```python
from build123d import *

# Parameters (mm, degrees)
F0_W           = 20.32
F0_H           = 12.7
F1_DEPTH       = 37.084
F5_D           = 9.525
F5_DEPTH       = 6.35
F5_TIP         = 2.8615986981
F5_ON_F3_D     = 9.525
F5_ON_F3_DEPTH = 6.35
F5_ON_F3_TIP   = 2.8615986981
F5_ON_F4_D     = 9.525
F5_ON_F4_DEPTH = 6.35
F5_ON_F4_TIP   = 2.8615986981
F7_DEPTH       = 37.085
F8_R           = 5.08


# Not quite as in the source:
# - a length typed as a fraction of an inch, garbled in the dataset ("3 / 203.2 mm" for 3/8 in), is restored


with BuildPart() as f1:
    # F0 (on Top) → F1 (new body)
    with BuildSketch(Plane.XY):
        with Locations((58.5882579065, 69.85)):
            Rectangle(F0_W, F0_H)
        Polygon((48.4282579065, 63.5), (-36.6617420935, 63.5), (0, 0), (117.1765158129, 0), (153.8382579065, 63.5), (68.7482579065, 63.5), align=None)
    extrude(amount=F1_DEPTH)

    # F5
    with Locations(Plane(origin=(0, 63.5, 0), x_dir=(-1, 0, 0), z_dir=(0, 1, 0))):
        with Locations((-136.8202579065, 18.542), (-119.8022579065, 18.542), (-102.7842579065, 18.542), (-85.7662579065, 18.542)):
            Hole(F5_D / 2, depth=F5_DEPTH)
            with Locations((0, 0, -(F5_DEPTH + F5_TIP / 2))):  # 118° drill point
                Cone(0, F5_D / 2, F5_TIP, mode=Mode.SUBTRACT)

    # F5 on F3
    with Locations(Plane(origin=(0, 63.5, 0), x_dir=(-1, 0, 0), z_dir=(0, 1, 0))):
        with Locations((-31.4102579065, 18.542), (-14.3922579065, 18.542), (2.6257420935, 18.542), (19.6437420935, 18.542)):
            Hole(F5_ON_F3_D / 2, depth=F5_ON_F3_DEPTH)
            with Locations((0, 0, -(F5_ON_F3_DEPTH + F5_ON_F3_TIP / 2))):  # 118° drill point
                Cone(0, F5_ON_F3_D / 2, F5_ON_F3_TIP, mode=Mode.SUBTRACT)

    # F5 on F4
    with Locations(Plane(origin=(0, 76.2, 0), x_dir=(-1, 0, 0), z_dir=(0, 1, 0))):
        with Locations((-58.5882579065, 18.542)):
            Hole(F5_ON_F4_D / 2, depth=F5_ON_F4_DEPTH)
            with Locations((0, 0, -(F5_ON_F4_DEPTH + F5_ON_F4_TIP / 2))):  # 118° drill point
                Cone(0, F5_ON_F4_D / 2, F5_ON_F4_TIP, mode=Mode.SUBTRACT)

    # F6 (on face) → F7 (cut, through all)
    with BuildSketch(Plane.XY.offset(37.084)):
        Polygon((26.8260418486, 48.1655448196), (-21.4583902673, 48.1655448196), (2.6838257906, 6.35), align=None)
        Polygon((54.7782579065, 6.35), (30.6360418486, 48.1655448196), (6.4938257906, 6.35), align=None)
        Polygon((82.7304739644, 48.1655448196), (34.4460418486, 48.1655448196), (58.5882579065, 6.35), align=None)
        Polygon((110.6826900223, 6.35), (86.5404739644, 48.1655448196), (62.3982579065, 6.35), align=None)
        Polygon((138.6349060802, 48.1655448196), (90.3504739644, 48.1655448196), (114.4926900223, 6.35), align=None)
    extrude(amount=-F7_DEPTH, mode=Mode.SUBTRACT)

    # F8
    f8_edges = [f1.edges().sort_by_distance(p)[0] for p in [
        (48.428258, 63.5, 18.542),
        (68.748258, 63.5, 18.542),
        (48.428258, 76.2, 18.542),
        (68.748258, 76.2, 18.542),
        (153.838258, 63.5, 18.542),
        (-36.661742, 63.5, 18.542),
        (-21.45839, 48.165545, 18.542),
        (0, 0, 18.542),
        (26.826042, 48.165545, 18.542),
        (82.730474, 48.165545, 18.542),
        (138.634906, 48.165545, 18.542),
        (110.68269, 6.35, 18.542),
        (114.49269, 6.35, 18.542),
        (2.683826, 6.35, 18.542),
        (117.176516, 0, 18.542),
        (90.350474, 48.165545, 18.542),
        (34.446042, 48.165545, 18.542),
        (30.636042, 48.165545, 18.542),
        (86.540474, 48.165545, 18.542),
        (62.398258, 6.35, 18.542),
        (6.493826, 6.35, 18.542),
        (58.588258, 6.35, 18.542),
        (54.778258, 6.35, 18.542),
    ]]
    fillet(f8_edges, radius=F8_R)


solid = f1.part
```
Here's how the part is built. I have some questions about the finished solid (model axes, mm). A direction names the side the tool comes from. Round coordinates to 2 decimals unless told otherwise and drop trailing zeros. Loops run counter-clockwise (first coordinate to the right, second up) from the corner with the lowest first, then second, coordinate; pieces in that order, holes last.
1. Thinking about a two-plate mould opening in Z: for faces 4 (the face through (58, 50, 0)), 5 (the face through (115.044, 60.281, 18.751)), 6 (the face through (14.648, 27.072, 18.802)), which applies, released by +Z, released by -Z, zero draft, split by the parting line, or undercut?
Answers:
face 4: released by -Z
face 5: undercut
face 6: zero draft
2. Suppose I cut it at C-C, the plane z = 5. Give the number of separate pieces and of enclosed holes in the cut face, and give its area (3 significant figures).
Answers:
separate pieces: 1
enclosed holes: 5
area: 5,210 mm2
3. Will these pins go through, and if not, where does the flat tip stop? pin 1 (11 mm diameter, centred on x = -5.5, z = 13.5, fed in from +Y); pin 2 (8 mm diameter, centred on y = 15, z = 19, fed in from +X); pin 3 (8.5 mm diameter, centred on x = -19.64, z = 18.54, fed in from -Y).
Answers:
pin 1: stops at y = 63.5
pin 2: stops at x = 128.15
pin 3: stops at y = 26.66
4. Suppose I cut it at A-A, the plane x = 127. Please give me the cut outline in (y, z), and give its area (3 significant figures).
Answers:
outline: (17.01, 0) - (28.01, 0) - (28.01, 37.08) - (17.01, 37.08) - close; (48.17, 0) - (63.5, 0) - (63.5, 37.08) - (48.17, 37.08) - close
area: 977 mm2
5. Suppose I cut it at D-D, the plane y = 51. Please give me the cut outline in (x, z).
Answers:
outline: (-29.44, 0) - (146.62, 0) - (146.62, 37.08) - (-29.44, 37.08) - close
6. Suppose I cut it at B-B, the plane y = 18. Please give me the cut outline in (x, z), and give its area (3 significant figures).
Answers:
outline: (-10.39, 0) - (-4.04, 0) - (-4.04, 37.08) - (-10.39, 37.08) - close; (9.41, 0) - (13.22, 0) - (13.22, 37.08) - (9.41, 37.08) - close; (48.05, 0) - (51.86, 0) - (51.86, 37.08) - (48.05, 37.08) - close; (65.31, 0) - (69.12, 0) - (69.12, 37.08) - (65.31, 37.08) - close; (103.96, 0) - (107.77, 0) - (107.77, 37.08) - (103.96, 37.08) - close; (121.22, 0) - (127.57, 0) - (127.57, 37.08) - (121.22, 37.08) - close
area: 1,040 mm2
7. If I drill on probe 1 along Y at (x, z) = (103, 3); probe 2 along X at (y, z) = (10.5, 14.5); probe 3 along X at (y, z) = (7, 27), over which ranges is the centre line in solid material (lowest first)?
Answers:
probe 1: y = 0 to 6.47, 19.66 to 26.26, 48.17 to 63.5
probe 2: x = -6.06 to 10.3, 50.97 to 66.2, 106.88 to 123.24
probe 3: x = -4.04 to 12.81, 48.47 to 68.71, 104.37 to 121.22
8. For faces 1 (the face through (3, 48.166, 19)), 2 (the face through (-3.658, 60.281, 13.893)), 3 (the face through (133.825, 28.837, 18.282)), which set-ups out of +Z, -Z, +X, -X, +Y, -Y let a thin tool reach every point of the face, with its end or its side?
Answers:
face 1: +Z, -Z
face 2: +Y
face 3: +Z, -Z, +X, -Y
